Autodesk Inventor part; units mm, degrees
ref_plane "YZ Plane" through (0, 0, 0) normal (1, 0, 0) x (0, 1, 0)
ref_plane "XZ Plane" through (0, 0, 0) normal (0, 1, 0) x (-1, 0, 0)
ref_plane "XY Plane" through (0, 0, 0) normal (0, 0, 1) x (1, 0, 0)
sketch "Sketch1" plane through (0, 0, 0) normal (1, 0, 0) x (0, 1, 0)
  line L0 (-6.35, 6.35) -> (6.35, 6.35)
  line L1 (6.35, 6.35) -> (6.35, -6.35)
  line L2 (6.35, -6.35) -> (-6.35, -6.35)
  line L3 (-6.35, -6.35) -> (-6.35, 6.35)
  line L4 (-6.35, 6.35) -> (6.35, -6.35) construction
  line L5 (6.35, 6.35) -> (-6.35, -6.35) construction
  line L6 (-4.35, 4.35) -> (4.35, 4.35)
  line L7 (4.35, 4.35) -> (4.35, -4.35)
  line L8 (4.35, -4.35) -> (-4.35, -4.35)
  line L9 (-4.35, -4.35) -> (-4.35, 4.35)
  line L10 (-4.35, 4.35) -> (4.35, -4.35) construction
  line L11 (4.35, 4.35) -> (-4.35, -4.35) construction
  point P0 (0, 0)
  dimension "d0" = 12.7
  dimension "d1" = 12.7
  dimension "d15" = 2
  dimension "d16" = 2
extrude "Extrusion1" add sketch "Sketch1" along normal mid plane 400
sketch "Sketch2" plane through (-200, 6.35, 6.35) normal (0, 1, 0) x (1, 0, 0)
  circle A0 centre (5, 6.35) radius 2.6
  line L0 (14, 6.35) -> (50, 6.35) construction
  line L1 (14, 3.75) -> (50, 3.75)
  line L2 (50, 8.95) -> (14, 8.95)
  arc A1 (14, 8.95) -> (14, 3.75) centre (14, 6.35) ccw
  arc A2 (50, 3.75) -> (50, 8.95) centre (50, 6.35) ccw
  line L3 (0, 0) -> (0, 12.7)
  circle A3 centre (118, 6.35) radius 2.6
  circle A4 centre (185, 6.35) radius 2.6
  point P0 (200, 6.35)
  point P1 (32, 6.35)
  dimension "d6" = 5.2
  dimension "d7" = 5
  dimension "d8" = 9
  dimension "d9" = 36
  dimension "d13" = 67
  dimension "d14" = 15
extrude "Extrusion2" cut sketch "Sketch2" against normal blind 100
mirror "Mirror1" about plane through (0, 0, 0) normal (1, 0, 0) of "Extrusion2"
properties part number "holder_bar"
Source: CAD feature listing. Evaluate the final solid. Frame: model axes, mm. A direction names the side the tool comes from. Coordinates: 2 decimals unless noted, no trailing zeros. Write each loop counter-clockwise with the first axis right and the second up, starting at its lowest first coordinate (ties: lowest second). Pieces come first, ordered by that corner, then holes. Notation, with made-up numbers: M 56.5,-1 L 107.5,-1 A15 cw 107.5,5 Z; hole C -36,88 d2. An arc over 180 degrees is marked long. Answer as a JSON object with one key per item and string values.
1. Access query for faces 1 (the flat face through (-3, -4.35, 0)), 2 (the flat face through (-3, -6.35, 0)). Directions: +Z, -Z, +X, -X, +Y, -Y. A direction counts if a zero-diameter tool reaches every point of the face in a straight line with its end or side. Return the directions, or none.
Evaluation:
{"face 1": "+X, -X", "face 2": "+Z, -Z, +X, -X, -Y"}
2. Cut plane B-B on x = 5.5. Output: boundary loops of the cut face in (y, z).
Evaluation:
{"outline": "M -6.35,-6.35 L 6.35,-6.35 L 6.35,6.35 L -6.35,6.35 Z; hole M -4.35,-4.35 L 4.35,-4.35 L 4.35,4.35 L -4.35,4.35 Z"}
3. Contact query for a flat-ended pin moving along its axis: P1, Ø4, axis at x = -82, z = 0, coming from the -Y side. Output: stop coordinate, or through.
Evaluation:
{"P1": "through"}
4. Cut plane A-A on x = -172. Output: boundary loops of the cut face in (y, z), plus the area to 3 significant figures.
Evaluation:
{"outline": "M -6.35,-6.35 L 6.35,-6.35 L 6.35,-2.6 L 4.35,-2.6 L 4.35,-4.35 L -4.35,-4.35 L -4.35,-2.6 L -6.35,-2.6 Z; M -6.35,2.6 L -4.35,2.6 L -4.35,4.35 L 4.35,4.35 L 4.35,2.6 L 6.35,2.6 L 6.35,6.35 L -6.35,6.35 Z", "area": "64.8 mm^2"}
5. Ray query, L1, parallel to Y at x = -156, z = 3.25; L2, parallel to Z at x = 195, y = -5.7. Return the intervals inside material, ascending.
Evaluation:
{"L1": "-6.35 to -4.35, 4.35 to 6.35", "L2": "-6.35 to -2.6, 2.6 to 6.35"}
6. Cut plane C-C on z = 0. State how many separate pieces and enclosed holes the cut face has, plus the area to 3 significant figures.
Evaluation:
{"separate pieces": "18", "enclosed holes": "0", "area": "1,150 mm^2"}
7. Draft query along Y for faces 3 (the flat face through (-3, 4.35, 0)), 4 (the flat face through (-3, 6.35, 0)), 5 (the flat face through (-3, 0, 6.35)). Return one class per face: released by +Y, released by -Y, zero draft, split by the parting line, or undercut.
Evaluation:
{"face 3": "undercut", "face 4": "released by +Y", "face 5": "zero draft"}
